The model under review builds one solid part; all positions refer to its coordinate system, in mm. Face numbers are marked on the shaded views. A direction names the side the tool comes from. Round coordinates to 2 decimals unless told otherwise and drop trailing zeros. Order: outer loops, then holes, each group sorted by start corner. A loop starts at its lowest first (then second) coordinate and runs counter-clockwise, first axis right, second up. Notation, with made-up numbers: M -15.5,67.25 L -8.5,67.25 A18 ccw -8.5,76.25 Z; hole C 52,81.25 d5. An arc over 180 degrees is marked long. Answer as a JSON object with one key per item and string values. Group by question number.
1) To check wall thickness, follow line 1 (X direction, y = 15.5, z = 16); line 2 (Y direction, x = -6.5, z = 14); line 3 (Y direction, x = -20.5, z = 22). State the ranges of each line that lie inside material, in increasing order.
2) For the marked faces 1, 2 and 3, list the 3-axis set-ups (+Z, -Z, +X, -X, +Y, -Y) from which the entire face can be reached by the end or side of a thin tool; tool diameter is ignored.
3) Consider section D-D, the plane y = -1.5. Write out the cut boundary in (x, z).
4) Consider section C-C, the plane z = 16.5. Write out the cut boundary in (x, y), then the cut area to 3 significant figures.
5) Consider section A-A, the plane y = 24. Write out the cut boundary in (x, z), then the cut area to 3 significant figures.
6) Consider section B-B, the plane x = -10. Write out the cut boundary in (y, z).
7) Insertion check: pin 1 Ø5 at (x, z) = (-7, 11.5) entering from -Y; pin 2 Ø12 at (x, y) = (-21, -4) entering from +Z; pin 3 Ø12 at (y, z) = (6.5, 7.5) entering from -X; pin 4 Ø1 at (y, z) = (6.5, 27) entering from +X. Each pin has a flat end and moves straight along its axis. Give the tip position at first contact, or say it passes through.
```python
from build123d import *

# Parameters (mm, degrees)
F1_DEPTH = 31.75
F3_DEPTH = 12.7
F5_DEPTH = 12.7
F7_DEPTH = 12.7


with BuildPart() as f1:
    # F0 (on Top) → F1 (new body)
    with BuildSketch(Plane.XY):
        Polygon((-12.7, 0), (0, 0), (0, 25.4), (12.7, 25.4), (12.7, 44.45), (-25.4, 44.45), (-25.4, 25.4), (-12.7, 25.4), align=None)
    extrude(amount=F1_DEPTH)

    # F2 (on face) → F3 (join)
    with BuildSketch(Plane.YZ):
        Polygon((25.4, 31.75), (14.131341, 0), (25.4, 0), align=None)
    extrude(amount=F3_DEPTH)

    # F4 (on face) → F5 (join)
    with BuildSketch(Plane(origin=(-12.7, 0, 0), x_dir=(0, -1, 0), z_dir=(-1, 0, 0))):
        Polygon((-25.4, 0), (-11.329167, 0), (-25.4, 31.75), align=None)
    extrude(amount=F5_DEPTH)

    # F6 (on face) → F7 (join)
    with BuildSketch(Plane.YZ):
        Polygon((0, 31.75), (0, 0), (14.131341, 0), (25.4, 31.75), align=None)
        Polygon((-12.7, 0), (0, 0), (0, 31.75), align=None)
    extrude(amount=-F7_DEPTH)


solid = f1.part
```
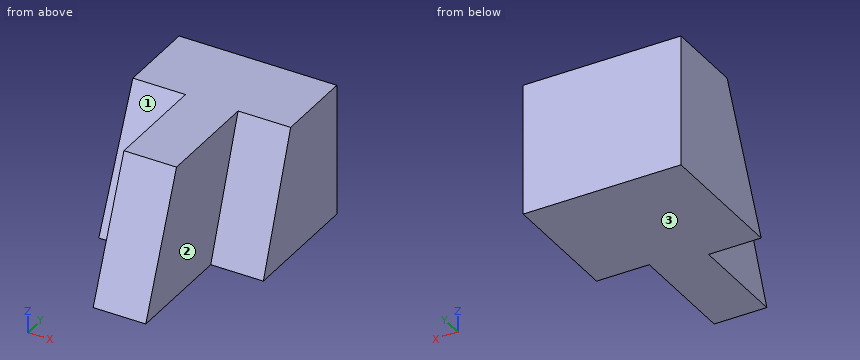
Results list:
{
 "1": {"line 1": "-12.7 to 0", "line 2": "-7.1 to 44.45", "line 3": "21.08 to 44.45"},
 "2": {"face 1": "+Z, -X, -Y", "face 2": "+Z, +X, -Y", "face 3": "-Z, +X, -X, +Y, -Y"},
 "3": {"outline": "M -12.7,0 L 0,0 L 0,28 L -12.7,28 Z"},
 "4": {"outline": "M -25.4,18.64 L -12.7,18.64 L -12.7,-6.1 L 0,-6.1 L 0,19.99 L 12.7,19.99 L 12.7,44.45 L -25.4,44.45 Z", "area": "1,280 mm^2"},
 "5": {"outline": "M -25.4,0 L 12.7,0 L 12.7,27.81 L 0,27.81 L 0,31.75 L -12.7,31.75 L -12.7,28.59 L -25.4,28.59 Z", "area": "1,120 mm^2"},
 "6": {"outline": "M -12.7,0 L 44.45,0 L 44.45,31.75 L 0,31.75 Z"},
 "7": {"pin 1": "y = -9.1", "pin 2": "through", "pin 3": "x = -12.7", "pin 4": "x = 0"}
}
